Drawing for the job (mm, zero at the part's lowest x, y, z). Round coordinates to 2 decimals unless told otherwise and drop trailing zeros. Order: outer loops, then holes, each group sorted by start corner. A loop starts at its lowest first (then second) coordinate and runs counter-clockwise, first axis right, second up. Notation, with made-up numbers: (-8.75, 43) - (49.25, 43) arc R7 ccw to (49.25, 51) - close; hole circle Ø8 at (54, 68). An arc over 180 degrees is marked (long way). Answer as a JSON object with one key per item and string values.
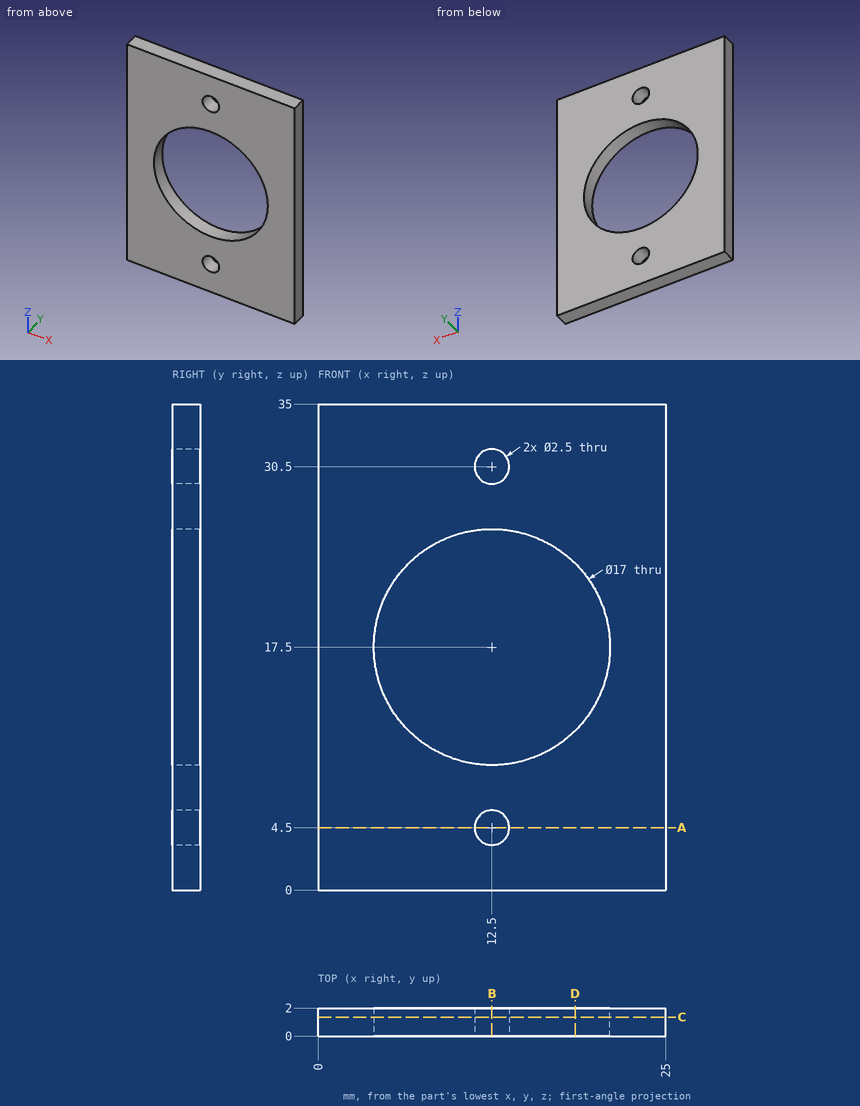
Item 1: Probe L1, parallel to Z at x = 12.5, y = 0.9; L2, parallel to X at y = 0.95, z = 4.5; L3, parallel to Z at x = 13, y = 1.35. List the from-to ranges inside material, lowest first. Write a range as from..to.
Taken from the geometry:
{"L1": "0..3.25, 5.75..9, 26..29.25, 31.75..35", "L2": "0..11.25, 13.75..25", "L3": "0..3.35, 5.65..9.01, 25.99..29.35, 31.65..35"}
Item 2: Cut at D-D (x = 18.5). Write the cut outline in (y, z), plus the area to 3 significant figures.
Taken from the geometry:
{"outline": "(0, 0) - (2, 0) - (2, 11.48) - (0, 11.48) - close; (0, 23.52) - (2, 23.52) - (2, 35) - (0, 35) - close", "area": "45.9 mm2"}
Item 3: Cut at C-C (y = 1.35). Write the cut outline in (x, z).
Taken from the geometry:
{"outline": "(0, 0) - (25, 0) - (25, 35) - (0, 35) - close; hole circle Ø17 at (12.5, 17.5); hole circle Ø2.5 at (12.5, 4.5); hole circle Ø2.5 at (12.5, 30.5)"}
Item 4: Cut at B-B (x = 12.5). Write the cut outline in (y, z), plus the area to 3 significant figures.
Taken from the geometry:
{"outline": "(0, 0) - (2, 0) - (2, 3.25) - (0, 3.25) - close; (0, 5.75) - (2, 5.75) - (2, 9) - (0, 9) - close; (0, 26) - (2, 26) - (2, 29.25) - (0, 29.25) - close; (0, 31.75) - (2, 31.75) - (2, 35) - (0, 35) - close", "area": "26.0 mm2"}
Item 5: Drop a flat-ended pin along its axis: P1, Ø3, axis at x = 12.5, z = 4.5, coming from the -Y side. Give the stop position or say it passes through.
Taken from the geometry:
{"P1": "y = 0"}
Item 6: Cut at A-A (z = 4.5). Write the cut outline in (x, y).
Taken from the geometry:
{"outline": "(0, 0) - (11.25, 0) - (11.25, 2) - (0, 2) - close; (13.75, 0) - (25, 0) - (25, 2) - (13.75, 2) - close"}
